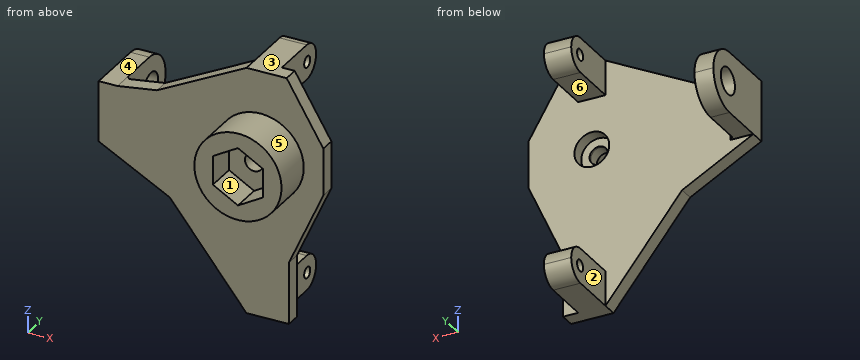
Autodesk Inventor part; units mm, degrees
ref_plane "YZ Plane" through (0, 0, 0) normal (1, 0, 0) x (0, 1, 0)
ref_plane "XZ Plane" through (0, 0, 0) normal (0, 1, 0) x (-1, 0, 0)
ref_plane "XY Plane" through (0, 0, 0) normal (0, 0, 1) x (1, 0, 0)
sketch "Sketch2" plane through (0, 0, 0) normal (0, 1, 0) x (-1, 0, 0)
  line L0 (2.5334, 16.1644) -> (0.0334, 16.1644)
  line L1 (0.0334, 16.1644) -> (0.0334, 24.1644)
  line L2 (0.0334, 24.1644) -> (2.5334, 24.1644)
  line L3 (2.5334, 24.1644) -> (2.5334, 16.1644)
  line L4 (-20.5666, -1.6356) -> (-16.9666, -1.6356)
  line L5 (-16.9666, -1.6356) -> (-16.9666, 2.9644)
  line L6 (-16.9666, 2.9644) -> (-20.5666, 2.9644)
  line L7 (-20.5666, 2.9644) -> (-20.5666, -1.6356)
  line L8 (-20.5666, 30.9644) -> (-16.9666, 30.9644)
  line L9 (-16.9666, 30.9644) -> (-16.9666, 26.3644)
  line L10 (-16.9666, 26.3644) -> (-20.5666, 26.3644)
  line L11 (-20.5666, 26.3644) -> (-20.5666, 30.9644)
  point P0 (0, 0)
  point P1 (-20.5666, 0.6644)
  point P2 (-20.5666, 28.6644)
  point P3 (0.0334, 20.1644)
  dimension "d4" = 4.6
  dimension "d5" = 3.6
  dimension "d6" = 2.5
  dimension "d7" = 8
  dimension "d8" = 28
  dimension "d9" = 8.5
  dimension "d59" = 20.6
extrude "Extrusion2" add sketch "Sketch2" along normal blind 8.5
sketch "Sketch3" plane through (0, 8.5, 0) normal (0, 1, 0) x (1, 0, 0)
  line L0 (-2.5334, -24.1644) -> (-0.0334, -24.1644)
  line L1 (-0.0334, -24.1644) -> (-0.0334, -16.1644)
  line L2 (-0.0334, -16.1644) -> (-2.5334, -16.1644)
  line L3 (-2.5334, -16.1644) -> (-2.5334, -24.1644)
  point P0 (0, 0)
extrude "Extrusion3" add sketch "Sketch3" along normal blind 1.4
fillet "Fillet1" radius 2.3 4 edges at (18.7666, 8.5, 30.9644) (18.7666, 8.5, 26.3644) (18.7666, 8.5, 2.9644) (18.7666, 8.5, -1.6356)
fillet "Fillet2" radius 4 2 edges at (-1.2834, 9.9, 24.1644) (-1.2834, 9.9, 16.1644)
sketch "Sketch4" plane through (-0.0334, 0, 24.1644) normal (1, 0, 0) x (0, 0, -1)
  line L0 (8, 0) -> (0, 0)
  line L1 (4, 0) -> (4, 9.2517) construction
  line L2 (-6.8, 0) -> (-2.2, 0) construction
  line L3 (25.8, 0) -> (21.2, 0) construction
  line L4 (-4.5, 0) -> (-4.5, 8.5) construction
  arc A0 (-2.2, 6.2) -> (-6.8, 6.2) centre (-4.5, 6.2) ccw construction
  line L5 (23.5, 0) -> (23.5, 8.5) construction
  circle A1 centre (4, 6.3) radius 1.75
  circle A2 centre (23.5, 6.3) radius 0.75
  circle A3 centre (-4.5, 6.3) radius 0.75
  point P0 (24.1644, 0)
  dimension "d17" = 3.5
  dimension "d19" = 1.5
  dimension "d20" = 1.5
  dimension "d21" = 6.3
  dimension "d22" = 6.3
  dimension "d23" = 6.3
extrude "Extrusion4" cut sketch "Sketch4" along normal through all both and the other way through all
sketch "Sketch5" plane through (0, 0, 0) normal (0, -1, 0) x (1, 0, 0)
  line L0 (-2.5334, 16.1644) -> (6.8584, 11.1365)
  line L1 (6.8584, 11.1365) -> (16.9666, -1.6356)
  line L2 (16.9666, -1.6356) -> (20.5666, -1.6356)
  line L3 (20.5666, -1.6356) -> (16.9666, -1.6356)
  line L4 (20.5666, -1.6356) -> (22.5666, -1.6356)
  line L5 (22.2666, 30.9644) -> (20.5666, 30.9644)
  line L6 (20.5666, 30.9644) -> (16.9666, 30.9644)
  line L7 (16.9666, 30.9644) -> (5.172, 24.9376)
  line L8 (5.172, 24.9376) -> (-0.0334, 24.1644)
  line L9 (-0.0334, 24.1644) -> (-2.5334, 24.1644)
  line L10 (-0.0334, 24.1644) -> (-2.5334, 24.1644)
  line L11 (-2.5334, 24.1644) -> (-2.5334, 16.1644)
  line L12 (22.2666, 30.9644) -> (27.1025, 22.846)
  line L13 (27.1025, 22.846) -> (27.1025, 16.6045)
  line L14 (27.1025, 16.6045) -> (22.5666, 6.5187)
  line L15 (22.5666, 6.5187) -> (22.5666, -1.6356)
  point P0 (0, 0)
  dimension "d26" = 2
extrude "Extrusion5" add sketch "Sketch5" along normal blind 2
sketch "Sketch7" plane through (0, -2, 0) normal (0, -1, 0) x (1, 0, 0)
  line L0 (16.9666, 2.9644) -> (20.5666, 2.9644)
  line L1 (18.7666, 2.9644) -> (18.7666, 26.3644) construction
  line L2 (20.5666, 26.3644) -> (16.9666, 26.3644)
  line L3 (18.7666, 15.8122) -> (15.4666, 17.7174)
  line L4 (15.4666, 17.7174) -> (15.4666, 21.5279)
  line L5 (15.4666, 21.5279) -> (18.7666, 23.4332)
  line L6 (18.7666, 23.4332) -> (22.0666, 21.5279)
  line L7 (22.0666, 21.5279) -> (22.0666, 17.7174)
  line L8 (22.0666, 17.7174) -> (18.7666, 15.8122)
  line L9 (20.5666, 29.4144) -> (20.5666, 27.9144) construction
  line L10 (20.5666, 29.5605) -> (16.9666, 27.9144) construction
  line L11 (16.9666, 27.9144) -> (16.9666, 29.4144) construction
  line L12 (20.5666, 26.7294) -> (15.111, 29.4144) construction
  line L13 (16.9666, 29.4144) -> (20.5666, 29.4144) construction
  circle A0 centre (18.7666, 19.6227) radius 5.75
  point P0 (0, 0)
  point P1 (17.8388, 28.0719)
  dimension "d29" = 8.5
  dimension "d30" = 6.6
  dimension "d31" = 11.5
extrude "Extrusion6" add sketch "Sketch7" along normal blind 5.5
chamfer "Chamfer1" distance 0.5 angle 45 1 edges at (-0.0334, 0, 20.1644)
hole "Hole1" at (18.7666, 0, 19.6227) direction (0, -1, 0) diameter 2.4 end through all
hole "Hole2" at (18.7666, 0, 19.6227) direction (0, -1, 0) diameter 4.6 depth 1.7
sketch "Sketch8" plane through (0, -2, 0) normal (0, -1, 0) x (1, 0, 0)
  line L0 (18.7666, 23.4332) -> (22.0666, 21.5279)
  line L1 (22.0666, 21.5279) -> (22.0666, 17.7174)
  line L2 (22.0666, 17.7174) -> (18.7666, 15.8122)
  line L3 (18.7666, 15.8122) -> (15.4666, 17.7174)
  line L4 (15.4666, 17.7174) -> (15.4666, 21.5279)
  line L5 (15.4666, 21.5279) -> (18.7666, 23.4332)
  circle A0 centre (18.7666, 19.6227) radius 1.2
  point P0 (0, 0)
extrude "Extrusion7" add sketch "Sketch8" along normal blind 1.5
properties part number "servo_gimbal_interpart_1" material "ABS Plastic"
For this review, take the finished solid that the model builds, in its own axes (mm). Face numbers are marked on the shaded views. A direction names the side the tool comes from. Coordinates: 2 decimals unless noted, no trailing zeros. Order: outer loops, then holes, each group sorted by start corner. A loop starts at its lowest first (then second) coordinate and runs counter-clockwise, first axis right, second up. Notation, with made-up numbers: (-35, -38.5) -> (13, -38.5) arc R28 cw to (13, -13.5) -> close; hole circle Ø7 at (52.5, 47.25). An arc over 180 degrees is marked (long way). Answer as CSV lines item,"result".
Q1. We need section D-D (x = 5.75). State the section outline as (y, z) points, plus the area to 3 significant figures.
Model answer:
outline,"(-2, 11.73) -> (0, 11.73) -> (0, 25.23) -> (-2, 25.23) -> close"
area,"27.0 mm2"
Q2. Draft analysis for pull direction X (two halves, no side actions). For the marked faces 1, 2 and 3, state which applies: released by +X, released by -X, zero draft, split by the parting line, or undercut.
Model answer:
face 1,"undercut"
face 2,"released by -X"
face 3,"zero draft"
Q3. For the marked faces 4, 5 and 6, list the 3-axis set-ups (+Z, -Z, +X, -X, +Y, -Y) from which the entire face can be reached by the end or side of a thin tool; tool diameter is ignored.
Model answer:
face 4,"+Z, -X, +Y, -Y"
face 5,"-Y"
face 6,"+X, -X, +Y"
Q4. Clearance check with flat-ended pins moving along their axes: pin 1 Ø2 at (y, z) = (-0.5, 2) entering from +X; pin 2 Ø1.9 at (y, z) = (-5, 20.5) entering from +X; pin 3 Ø3 at (x, z) = (7, 24) entering from +Y. State where each tip first meets the part, or that it passes through.
Model answer:
pin 1,"stops at x = 22.57"
pin 2,"stops at x = 24.52"
pin 3,"stops at y = 0"
Q5. We need section B-B (y = -4). State the section outline as (x, z) points, plus the area to 3 significant figures.
Model answer:
outline,"circle Ø11.5 at (18.77, 19.62); hole (15.47, 17.72) -> (18.77, 15.81) -> (22.07, 17.72) -> (22.07, 21.53) -> (18.77, 23.43) -> (15.47, 21.53) -> close"
area,"66.1 mm2"
Q6. We need section C-C (z = 13). State the section outline as (x, y) points, plus the area to 3 significant figures.
Model answer:
outline,"(3.38, -2) -> (25.48, -2) -> (25.48, 0) -> (3.38, 0) -> close"
area,"44.2 mm2"
Q7. Wall thickness on line 1 along Z through (x, y) = (19.3, 6.3); line 2 along Z through (x, y) = (18.25, 1.25); line 3 along Y through (x, z) = (19, 24.5): over which ranges is each line inside the solid? List them lowest first. Write a range as [from, to].
Model answer:
line 1,"z = [-1.63, -0.09], [1.41, 2.96], [26.37, 27.91], [29.41, 30.96]"
line 2,"z = [-1.64, 2.96], [26.36, 30.96]"
line 3,"y = [-7.5, 0]"
Q8. We need section A-A (y = 2). State the section outline as (x, z) points.
Model answer:
outline,"(-2.53, 16.16) -> (-0.03, 16.16) -> (-0.03, 24.16) -> (-2.53, 24.16) -> close; (16.97, -1.64) -> (20.57, -1.64) -> (20.57, 2.96) -> (16.97, 2.96) -> close; (16.97, 26.36) -> (20.57, 26.36) -> (20.57, 30.96) -> (16.97, 30.96) -> close"
